from build123d import *

# Parameters (mm, degrees)
SKETCH1_R                                           = 6.35
BOSS_EXTRUDE1_DEPTH                                 = 3.175
SKETCH5_R                                           = 0.1905
CUT_EXTRUDE3_DEPTH                                  = 1.905
CIRPATTERN3_COUNT                                   = 3
SKETCH6_R                                           = 0.8509
CUT_EXTRUDE4_DEPTH                                  = 3.175
CBORE_FOR_2_BINDING_HEAD_MACHINE_SCREW1_D           = 2.1844
CBORE_FOR_2_BINDING_HEAD_MACHINE_SCREW1_CBORE_D     = 4.2418
CBORE_FOR_2_BINDING_HEAD_MACHINE_SCREW1_CBORE_DEPTH = 1.524
CIRPATTERN4_COUNT                                   = 3


with BuildPart() as part:
    # Sketch1 → Boss-Extrude1 (new body)
    with BuildSketch(Plane(origin=(0, 0, 0), x_dir=(1, 0, 0), z_dir=(0, 1, 0))):
        with Locations(Location((0, 0, 0), (0, 0, 270))):
            Circle(SKETCH1_R)
    extrude(amount=BOSS_EXTRUDE1_DEPTH)

    # Sketch5 → Cut-Extrude3 (cut)
    with BuildSketch(Plane(origin=(0, 3.175, 0), x_dir=(1, 0, 0), z_dir=(0, 1, 0))):
        with Locations(Location((0, 1.778, 0), (0, 0, 270))):
            Circle(SKETCH5_R)
    cut_extrude3 = extrude(amount=-CUT_EXTRUDE3_DEPTH, mode=Mode.SUBTRACT)

    # CirPattern3: Cut-Extrude3 ×3 about axis
    cirpattern3_axis = Axis((0, 0, 0), (0, 1, 0))
    for i in range(1, CIRPATTERN3_COUNT):
        add(cut_extrude3.rotate(cirpattern3_axis, i * 360 / CIRPATTERN3_COUNT), mode=Mode.SUBTRACT)

    # Sketch6 → Cut-Extrude4 (cut)
    with BuildSketch(Plane(origin=(0, 3.175, 0), x_dir=(1, 0, 0), z_dir=(0, 1, 0))):
        with Locations(Location((0, 0, 0), (0, 0, 270))):
            Circle(SKETCH6_R)
    extrude(amount=-CUT_EXTRUDE4_DEPTH, mode=Mode.SUBTRACT)

    # CBORE for #2 Binding Head Machine Screw1 (through all)
    with Locations(Plane(origin=(0, 3.175, 0), x_dir=(1, 0, 0), z_dir=(0, 1, 0))):
        with Locations((0, -3.81)):
            cbore_for_2_binding_head_machine_screw1 = CounterBoreHole(CBORE_FOR_2_BINDING_HEAD_MACHINE_SCREW1_D / 2, CBORE_FOR_2_BINDING_HEAD_MACHINE_SCREW1_CBORE_D / 2, CBORE_FOR_2_BINDING_HEAD_MACHINE_SCREW1_CBORE_DEPTH)

    # CirPattern4: CBORE for #2 Binding Head Machine Screw1 ×3 about axis
    cirpattern4_axis = Axis((0, 0, 0), (0, 1, 0))
    for i in range(1, CIRPATTERN4_COUNT):
        add(cbore_for_2_binding_head_machine_screw1.rotate(cirpattern4_axis, i * 360 / CIRPATTERN4_COUNT), mode=Mode.SUBTRACT)


solid = part.part
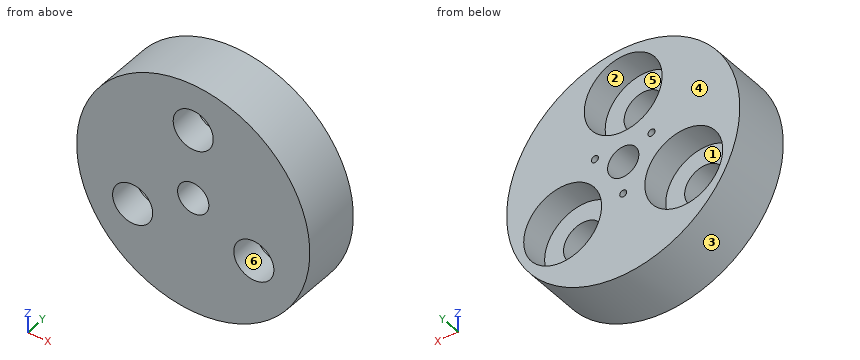
Work out the finished part from the listing and answer in its coordinate system (mm). Face numbers are marked on the shaded views. A direction names the side the tool comes from. Coordinates: 2 decimals unless noted, no trailing zeros. Write each loop counter-clockwise with the first axis right and the second up, starting at its lowest first coordinate (ties: lowest second). Pieces come first, ordered by that corner, then holes. Notation, with made-up numbers: M 14,11.25 L 58,11.25 A18 cw 58,35.25 Z; hole C 7,77.5 d1. An arc over 180 degrees is marked long. Answer as CSV lines item,"result". Start each with the question number.
Item 1: Flat-ended cylindrical pins translate along their axes: P1, Ø2, axis at x = 0, z = 0, coming from the -Y side; P2, Ø3.5, axis at x = 0, z = 3.81, coming from the +Y side. Find the tip coordinate at first contact, or state that the pin passes through.
Item 2: Section C-C on x = 3.5 is taken. Write down the section's boundary in (y, z) (3 decimals).
Item 3: Consider L1, parallel to X at y = 2.55, z = -2.25; L2, parallel to Y at x = -2.5, z = -0.5; L3, parallel to Z at x = 0.75, y = 1.8. Determine where each line is inside the solid, lowest interval first.
Item 4: Section B-B on x = 0 is taken. Give the number of separate pieces and of enclosed holes in the cut face, and give its area (3 significant figures).
Item 5: Section A-A on z = 3.81 is taken. Write down the section's boundary in (x, y) (3 decimals), and give its area (3 significant figures).
Item 6: A tool of negligible diameter and unlimited length cuts with its end or side. For the marked faces 5 and 6, from which of +Z, -Z, +X, -X, +Y, -Y can it reach the whole face along a straight path? Write none if from no direction.
Item 7: Determine the mould class of the marked faces 1, 2, 3 and 4 for opening direction X: released by +X, released by -X, zero draft, split by the parting line, or undercut.
Checks:
1,P1,"stops at y = 0"
1,P2,"stops at y = 1.65"
2,outline,"M 0,-5.298 L 3.175,-5.298 L 3.175,-4.016 L 1.651,-4.016 L 1.651,-2.979 L 0,-2.979 Z; M 0,-0.831 L 1.651,-0.831 L 1.651,0.206 L 3.175,0.206 L 3.175,5.298 L 0,5.298 Z"
3,L1,"x = -5.94 to -5.39, -1.21 to 1.21, 5.39 to 5.94"
3,L2,"y = 0 to 1.65"
3,L3,"z = -6.31 to -0.4, 0.4 to 1.83, 5.79 to 6.31"
4,separate pieces,"3"
4,enclosed holes,"0"
4,area,"24.1 mm²"
5,outline,"M -5.08,0 L -1.092,0 L -1.092,1.651 L -2.121,1.651 L -2.121,3.175 L -5.08,3.175 Z; M 1.092,0 L 5.08,0 L 5.08,3.175 L 2.121,3.175 L 2.121,1.651 L 1.092,1.651 Z"
5,area,"22.2 mm²"
6,face 5,"+Y"
6,face 6,"+Y, -Y"
7,face 1,"undercut"
7,face 2,"undercut"
7,face 3,"split by the parting line"
7,face 4,"zero draft"
